Build history of the part. All positions in model axes, mm. Face numbers are marked on the shaded views. A direction names the side the tool comes from. Coordinates: 2 decimals unless noted, no trailing zeros. Order: outer loops, then holes, each group sorted by start corner. A loop starts at its lowest first (then second) coordinate and runs counter-clockwise, first axis right, second up. Notation, with made-up numbers: M -5.75,43.25 L 35.25,43.25 A24 ccw 35.25,64.25 Z; hole C 77.5,-36 d7. An arc over 180 degrees is marked long. Use a Markdown table: item, result. Add a question column.
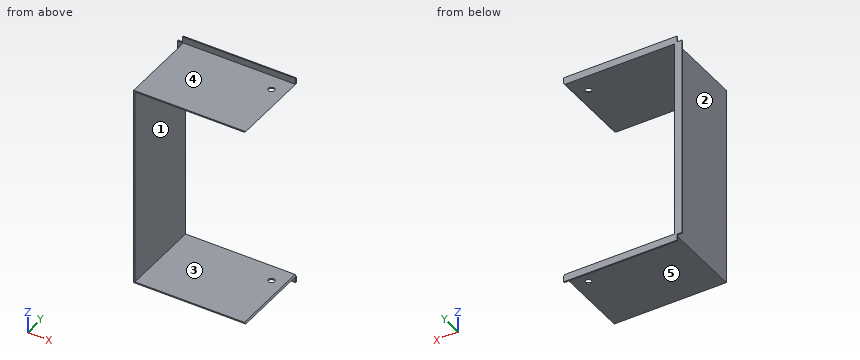
Autodesk Inventor part; units mm, degrees
ref_plane "YZ Plane" through (0, 0, 0) normal (1, 0, 0) x (0, 1, 0)
ref_plane "XZ Plane" through (0, 0, 0) normal (0, 1, 0) x (-1, 0, 0)
ref_plane "XY Plane" through (0, 0, 0) normal (0, 0, 1) x (1, 0, 0)
sketch "Sketch1" plane through (0, 0, 0) normal (0, 1, 0) x (-1, 0, 0)
  line L0 (-115.8875, -209.55) -> (115.8875, -209.55)
  line L1 (115.8875, -209.55) -> (115.8875, 209.55)
  line L2 (115.8875, 209.55) -> (-115.8875, 209.55)
  line L3 (-115.8875, -209.55) -> (115.8875, 209.55) construction
  line L4 (115.8875, -209.55) -> (-115.8875, 209.55) construction
  line L5 (113.3475, 207.01) -> (113.3475, -207.01)
  line L6 (113.3475, -207.01) -> (-113.3475, -207.01)
  line L7 (-113.3475, 207.01) -> (113.3475, 207.01)
  line L8 (-113.3475, 207.01) -> (-115.8875, 209.55)
  line L9 (-113.3475, -207.01) -> (-115.8875, -209.55)
  point P0 (0, 0)
  dimension "d0" = 231.775
  dimension "d1" = 419.1
  dimension "d2" = 2.54
extrude "Extrusion1" add sketch "Sketch1" along normal blind 127
sketch "Sketch2" plane through (0, 127, 0) normal (0, 1, 0) x (1, 0, 0)
  line L0 (-115.8875, -209.55) -> (-128.5875, -209.55)
  line L1 (-128.5875, -209.55) -> (-128.5875, 209.55)
  line L2 (-128.5875, 209.55) -> (-115.8875, 209.55)
  line L3 (-115.8875, 209.55) -> (-115.8875, -209.55)
  line L4 (-115.8875, 209.55) -> (115.8875, 209.55)
  line L5 (115.8875, 209.55) -> (115.8875, 222.25)
  line L6 (115.8875, 222.25) -> (-115.8875, 222.25)
  line L7 (-115.8875, 222.25) -> (-115.8875, 209.55)
  line L8 (-115.8875, -209.55) -> (115.8875, -209.55)
  line L9 (115.8875, -209.55) -> (-115.8875, -209.55)
  line L10 (-115.8875, -209.55) -> (-115.8875, -222.25)
  line L11 (-115.8875, -222.25) -> (115.8875, -222.25)
  line L12 (115.8875, -222.25) -> (115.8875, -209.55)
  point P0 (0, 0)
  dimension "d5" = 12.7
  dimension "d6" = 419.1
  dimension "d7" = 231.775
  dimension "d8" = 12.7
  dimension "d9" = 12.7
  dimension "d12" = 231.775
extrude "Extrusion2" add sketch "Sketch2" against normal blind 2.54
sketch "Sketch3" plane through (0, 0, 0) normal (0, -1, 0) x (1, 0, 0)
  line L0 (115.8875, -209.55) -> (-115.8875, -209.55)
  line L1 (113.3475, -207.01) -> (115.8875, -209.55)
  line L2 (-113.3475, -207.01) -> (113.3475, -207.01)
  line L3 (-113.3475, 207.01) -> (-113.3475, -207.01)
  line L4 (113.3475, 207.01) -> (-113.3475, 207.01)
  line L5 (115.8875, 209.55) -> (113.3475, 207.01)
  line L6 (-115.8875, 209.55) -> (115.8875, 209.55)
  line L7 (-115.8875, -209.55) -> (-115.8875, 209.55)
  point P0 (0, 0)
extrude "Extrusion3" add sketch "Sketch3" along normal blind 40.64
sketch "Sketch4" plane through (115.8875, 124.46, -209.55) normal (0, 0, -1) x (-1, 0, 0)
  circle A0 centre (27.94, -34.925) radius 6.35
  line L0 (0, 0) -> (0, -165.1)
  line L1 (231.775, 0) -> (0, 0)
  circle A1 centre (85.3615, -107.95) radius 99.06 construction
  point P0 (115.8875, -124.46)
  dimension "d15" = 12.7
  dimension "d25" = 27.94
  dimension "d26" = 34.925
extrude "Extrusion4" cut sketch "Sketch4" against normal through all
sketch "Sketch5" plane through (-115.8875, 127, -209.55) normal (0, 0, -1) x (-1, 0, 0)
  line L0 (5.08, -2.54) -> (5.08, 49.46)
  line L1 (0, 0) -> (0, -2.54)
  line L2 (2.54, -2.54) -> (2.54, -27.94)
  line L3 (0, -2.54) -> (0, 0)
  line L4 (0, 0) -> (2.54, 0)
  line L5 (2.54, 0) -> (2.54, -2.54)
  line L6 (2.54, -2.54) -> (0, -2.54)
  line L7 (0, -2.54) -> (0, 0)
  point P0 (-115.8875, -127)
extrude "Extrusion5" add sketch "Sketch5" along normal blind 12.7
sketch "Sketch6" plane through (0, 127, 0) normal (0, 1, 0) x (1, 0, 0)
  line L0 (-115.8875, -209.55) -> (-128.5875, -209.55)
  line L1 (-115.8875, -209.55) -> (-118.4275, -209.55)
  line L2 (-118.4275, -209.55) -> (-118.4275, -222.25)
  line L3 (-118.4275, -222.25) -> (-115.8875, -222.25)
  line L4 (-115.8875, -222.25) -> (-115.8875, -209.55)
  point P0 (0, 0)
  dimension "d20" = 2.54
extrude "Extrusion6" add sketch "Sketch6" against normal blind 2.54
properties part number "Intake Drop" material "Aluminum 6061"
(1) Drop flat-ended pins along their axis: P1, Ø3, axis at x = -122.5, y = 125.5, coming from the +Z side; P2, Ø4, axis at x = -45.5, y = -6, coming from the -Z side; P3, Ø1.5, axis at y = 14, z = -37, coming from the +X side. Give the stop position or say it passes through.
(2) Mould opens along Z. For the marked faces 3, 4 and 5 say: released by +Z, released by -Z, zero draft, split by the parting line, or undercut.
(3) Which spindle directions (+Z, -Z, +X, -X, +Y, -Y) get a long thin tool onto all of the face, cutting with end or side? Do the marked faces 1 and 2. Say none if no direction does.
(4) Slice it at A-A on x = 37. Give the cut face in (y, z), and give its area (3 significant figures).
(5) Drill centre lines: line 1 along Z through (x, y) = (92, 81); line 2 along X through (y, z) = (-17, -93). Where is each one in solid material? Low to high. Write a range as from..to.
(6) Slice it at B-B on y = 106.5. Give the cut face in (x, z), and give its area (3 significant figures).
(7) Slice it at C-C on z = -158. Give the cut face in (x, y), and give its area (3 significant figures).
Solutions:
| question | item | result |
|---|---|---|
| 1 | P1 | z = 209.55 |
| 1 | P2 | z = -209.55 |
| 1 | P3 | x = -113.35 |
| 2 | face 3 | undercut |
| 2 | face 4 | released by +Z |
| 2 | face 5 | released by -Z |
| 3 | face 1 | +X, +Y, -Y |
| 3 | face 2 | +Z, -Z, -X, -Y |
| 4 | outline | M -40.64,-209.55 L 124.46,-209.55 L 124.46,-222.25 L 127,-222.25 L 127,-207.01 L -40.64,-207.01 Z; M -40.64,207.01 L 127,207.01 L 127,222.25 L 124.46,222.25 L 124.46,209.55 L -40.64,209.55 Z |
| 4 | area | 916 mm² |
| 5 | line 1 | -209.55..-207.01, 207.01..209.55 |
| 5 | line 2 | -115.89..-113.35 |
| 6 | outline | M -115.89,-209.55 L 115.89,-209.55 L 113.35,-207.01 L -113.35,-207.01 L -113.35,207.01 L 113.35,207.01 L 115.89,209.55 L -115.89,209.55 Z |
| 6 | area | 2,220 mm² |
| 7 | outline | M -128.59,124.46 L -115.89,124.46 L -115.89,-40.64 L -113.35,-40.64 L -113.35,127 L -128.59,127 Z |
| 7 | area | 458 mm² |
